Build history of the part. All positions in model axes, mm. Face numbers are marked on the shaded views. Coordinates: 2 decimals unless noted, no trailing zeros. Loops run counter-clockwise (first coordinate to the right, second up) from the corner with the lowest first, then second, coordinate; pieces in that order, holes last.
(1) Two-plate mould, pull along Z, no slides. Class the marked faces 1, 2 and 3: pulls with the +Z half, pulls with the -Z half, needs draft (parallel to the pull), parting line crosses it, or undercut.
(2) Slice it at C-C (y = 18). Give the cut face in (x, z) (3 decimals), and give its area (3 significant figures).
(3) Slice it at D-D (x = -25.4). Give the cut face in (y, z) (3 decimals).
(4) Flat gauge pins, fed straight in: P1, Ø5, axis at y = 37, z = 46, coming from the +X side; P2, Ø1, axis at x = -31.5, y = 21.5, coming from the +Z side; P3, Ø15.5, axis at x = -25.4, z = 43.99, coming from the +Y side (3 decimals); P4, Ø1, axis at y = 16.5, z = 10.5, coming from the -X side. Where does each tip first touch, or does it go through?
(5) Wall check: L1, parallel to Z at x = 25, y = 2; L2, parallel to Z at x = 50.8, y = 1.7; L3, parallel to X at y = 27.5, z = -0.5. Give the ranges that are in metal, low to high.
(6) Slice it at A-A (z = 0). Give the cut face in (x, y) (3 decimals).
(7) Slice it at B-B (x = 50.8). Give the cut face in (y, z) (3 decimals), and give its area (3 significant figures).
from build123d import *

# Parameters (mm, degrees)
SKETCH3_R          = 6
CUT_EXTRUDE1_DEPTH = 102.649597269
CIRPATTERN1_COUNT  = 6


with BuildPart() as part:
    # Sketch1 → Revolve1 (revolve)
    with BuildSketch(Plane.XY, mode=Mode.PRIVATE) as revolve1_sk:
        Polygon((-63.5, 0), (-63.5, 3.175), (-41.275, 3.175), (-41.275, 50.8), (-38.1, 50.8), (-38.1, 0), align=None)
    revolve(revolve1_sk.sketch.rotate(Axis((0, 0, 0), (0, 1, 0)), 270), axis=Axis((0, 0, 0), (0, 1, 0)))

    # Sketch3 → Cut-Extrude1 (cut, symmetric)
    with BuildSketch(Plane(origin=(0, 3.175, 0), x_dir=(1, 0, 0), z_dir=(0, 1, 0))):
        with Locations(Location((-50.8, 0, 0), (0, 0, 270))):
            Circle(SKETCH3_R)
    cut_extrude1 = extrude(amount=CUT_EXTRUDE1_DEPTH, both=True, mode=Mode.SUBTRACT)

    # CirPattern1: Cut-Extrude1 ×6 about axis
    cirpattern1_axis = Axis((0, 0, 0), (0, 1, 0))
    for i in range(1, CIRPATTERN1_COUNT):
        add(cut_extrude1.rotate(cirpattern1_axis, i * 360 / CIRPATTERN1_COUNT), mode=Mode.SUBTRACT)


solid = part.part
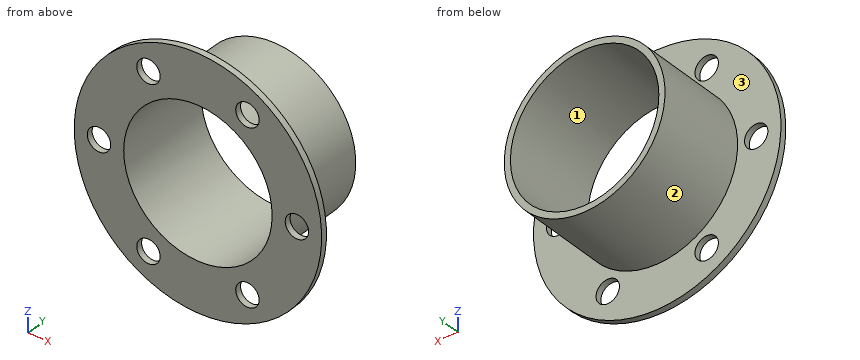
Response values:
1. face 1: undercut
1. face 2: parting line crosses it
1. face 3: needs draft
2. outline: circle Ø82.55 at (0, 0); hole circle Ø76.2 at (0, 0)
2. area: 792 mm2
3. outline: (0, -58.199) - (3.175, -58.199) - (3.175, -49.994) - (0, -49.994) - close; (0, -37.994) - (3.175, -37.994) - (3.175, -32.534) - (50.8, -32.534) - (50.8, -28.398) - (0, -28.398) - close; (0, 28.398) - (50.8, 28.398) - (50.8, 32.534) - (3.175, 32.534) - (3.175, 37.994) - (0, 37.994) - close; (0, 49.994) - (3.175, 49.994) - (3.175, 58.199) - (0, 58.199) - close
4. P1: passes through
4. P2: stops at z = 27.25
4. P3: stops at y = 3.175
4. P4: stops at x = -40.05
5. L1: z = -58.37 to -49.98, -38.01 to -28.75, 28.75 to 38.01, 49.98 to 58.37
5. L2: z = -38.1 to -6, 6 to 38.1
5. L3: x = -41.27 to -38.1, 38.1 to 41.27
6. outline: (-63.5, 0) - (-56.8, 0) - (-56.8, 3.175) - (-63.5, 3.175) - close; (-44.8, 0) - (-38.1, 0) - (-38.1, 50.8) - (-41.275, 50.8) - (-41.275, 3.175) - (-44.8, 3.175) - close; (38.1, 0) - (44.8, 0) - (44.8, 3.175) - (41.275, 3.175) - (41.275, 50.8) - (38.1, 50.8) - close; (56.8, 0) - (63.5, 0) - (63.5, 3.175) - (56.8, 3.175) - close
7. outline: (0, -38.1) - (3.175, -38.1) - (3.175, -6) - (0, -6) - close; (0, 6) - (3.175, 6) - (3.175, 38.1) - (0, 38.1) - close
7. area: 204 mm2
